Autodesk Inventor part; units mm, degrees
ref_plane "YZ Plane" through (0, 0, 0) normal (1, 0, 0) x (0, 1, 0)
ref_plane "XZ Plane" through (0, 0, 0) normal (0, 1, 0) x (-1, 0, 0)
ref_plane "XY Plane" through (0, 0, 0) normal (0, 0, 1) x (1, 0, 0)
sketch "Sketch1" plane through (0, 0, 0) normal (0, 0, 1) x (1, 0, 0)
  line L0 (0, 88.2) -> (0, -88.2)
  line L1 (-70, 0) -> (70, 0)
  line L2 (-50, -63) -> (50, -63)
  line L3 (50, -63) -> (50, 63)
  line L4 (50, 63) -> (-50, 63)
  line L5 (-50, 63) -> (-50, -63)
  circle A0 centre (0, -20) radius 30
  circle A1 centre (-30, 43) radius 4
  circle A2 centre (30, 43) radius 4
  circle A3 centre (34.8, -54.8) radius 3.25
  circle A4 centre (34.8, 14.8) radius 3.25
  circle A5 centre (-34.8, 14.8) radius 3.25
  circle A6 centre (-34.8, -54.8) radius 3.25
  line L6 (-30, 43) -> (-30, 39)
  line L7 (0, -20) -> (0, 10)
  point P0 (0, 0)
  dimension "d2" = 60
  dimension "d4" = 8
  dimension "d0" = 100
  dimension "d1" = 126
  dimension "d3" = 43
  dimension "d5" = 8
  dimension "d6" = 20
  dimension "d7" = 20
  dimension "d8" = 20
  dimension "d9" = 20
  dimension "d10" = 6.5
  dimension "d11" = 6.5
  dimension "d12" = 6.5
  dimension "d13" = 6.5
  dimension "d14" = 69.6
  dimension "d15" = 69.6
  dimension "d16" = 69.6
  dimension "d17" = 69.6
  dimension "d18" = 0
  dimension "d19" = 0
  dimension "d20" = 34.8
  dimension "d21" = 34.8
  dimension "d22" = 29
extrude "Extrusion1" add sketch "Sketch1" along normal blind 20 contours L4 L3 L1 A0 L0 | L0 A0 L1 L5 L4 | L1 L3 L2 L0 A0 | A0 L0 L2 L5 L1
sketch "Sketch2" plane through (0, 0, 20) normal (0, 0, 1) x (1, 0, 0)
  line L0 (50, 63) -> (-50, 63)
  line L1 (-50, 63) -> (-50, -63)
  line L2 (-50, -63) -> (50, -63)
  line L3 (50, -63) -> (50, 63)
  circle A0 centre (30, 43) radius 4
  circle A1 centre (34.8, 14.8) radius 3.25
  circle A2 centre (34.8, -54.8) radius 3.25
  circle A3 centre (-34.8, -54.8) radius 3.25
  circle A4 centre (-34.8, 14.8) radius 3.25
  circle A5 centre (-30, 43) radius 4
  circle A6 centre (0, -20) radius 30
  line L4 (-50, 63) -> (-50, -63)
  line L5 (-50, 43) -> (50, 43)
  line L6 (-50, 47) -> (50, 47)
  line L7 (-50, 39) -> (50, 39)
  point P0 (0, 0)
  dimension "d25" = 4
  dimension "d26" = 4
extrude "Extrusion2" cut sketch "Sketch2" against normal blind 4 contours L3 L6 L1 L0 | L3 L2 L1 L7
sketch "Sketch3" plane through (0, 0, 0) normal (0, 0, -1) x (-1, 0, 0)
  line L0 (-50, 63) -> (50, 63)
  line L1 (-50, -63) -> (-50, 63)
  line L2 (50, -63) -> (-50, -63)
  line L3 (50, 63) -> (50, -63)
  circle A0 centre (-30, 43) radius 4
  circle A1 centre (-34.8, 14.8) radius 3.25
  circle A2 centre (-34.8, -54.8) radius 3.25
  circle A3 centre (34.8, -54.8) radius 3.25
  circle A4 centre (34.8, 14.8) radius 3.25
  circle A5 centre (30, 43) radius 4
  circle A6 centre (0, -20) radius 30
  point P0 (0, 0)
extrude "Extrusion3" cut sketch "Sketch3" against normal blind 6
properties part number "motor mount lower"
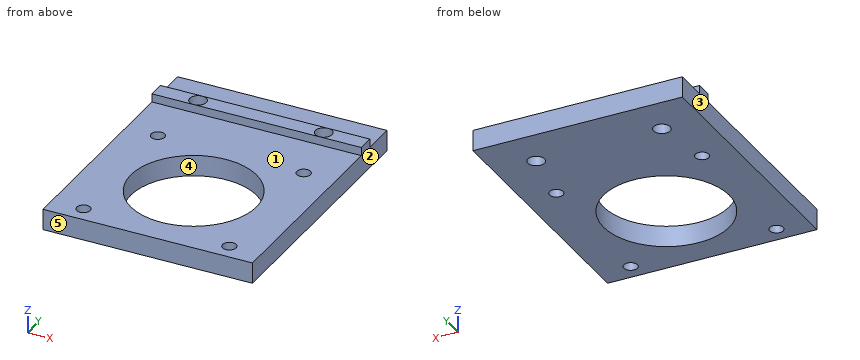
Model file for the job. Use its own axes, mm. Face numbers are marked on the shaded views. A direction names the side the tool comes from. Coordinates: 2 decimals unless noted, no trailing zeros. Write each loop counter-clockwise with the first axis right and the second up, starting at its lowest first coordinate (ties: lowest second). Pieces come first, ordered by that corner, then holes. Notation, with made-up numbers: (-14, 41) -> (44, 41) arc R19 ccw to (44, 78) -> close; hole circle Ø7 at (62, 33.5). An arc over 180 degrees is marked (long way). One line per item, written item: value. Start each with the question number.
1) Slice it at B-B on y = 14.8. Write the cut outline in (x, z), then the cut area to 3 significant figures.
2) Flat gauge pins, fed straight in: pin 1 Ø2 at (x, z) = (-14, 18) entering from -Y; pin 2 Ø6 at (x, y) = (-34.8, 14.8) entering from -Z; pin 3 Ø1.5 at (x, y) = (-10, 22.5) entering from +Z. Where does each tip first touch, or does it go through?
3) Slice it at A-A on z = 8. Write the cut outline in (x, y).
4) Slice it at D-D on y = -20. Write the cut outline in (x, z), then the cut area to 3 significant figures.
5) Slice it at C-C on x = 0. Write the cut outline in (y, z).
6) Pull direction X, two halves, no side cores. Call the marked faces 3, 4 and 5: +X half, -X half, draft (parallel to the pull), parting line (faces both ways), or undercut.
7) Which spindle directions (+Z, -Z, +X, -X, +Y, -Y) get a long thin tool onto all of the face, cutting with end or side? Do the marked faces 1 and 2. Say none if no direction does.
8) Probe probe 1 along Y at (x, z) = (34.8, 10.5); probe 2 along Y at (x, z) = (-27, 14.5); probe 3 along Y at (x, z) = (0, 10.5). List the from-to ranges inside material, lowest first.
Answers follow:
1. outline: (-50, 6) -> (-38.05, 6) -> (-38.05, 16) -> (-50, 16) -> close; (-31.55, 6) -> (31.55, 6) -> (31.55, 16) -> (-31.55, 16) -> close; (38.05, 6) -> (50, 6) -> (50, 16) -> (38.05, 16) -> close
1. area: 870 mm2
2. pin 1: y = 39
2. pin 2: through
2. pin 3: z = 16
3. outline: (-50, -63) -> (50, -63) -> (50, 63) -> (-50, 63) -> close; hole circle Ø6.5 at (-34.8, -54.8); hole circle Ø6.5 at (-34.8, 14.8); hole circle Ø8 at (-30, 43); hole circle Ø60 at (0, -20); hole circle Ø8 at (30, 43); hole circle Ø6.5 at (34.8, -54.8); hole circle Ø6.5 at (34.8, 14.8)
4. outline: (-50, 6) -> (-30, 6) -> (-30, 16) -> (-50, 16) -> close; (30, 6) -> (50, 6) -> (50, 16) -> (30, 16) -> close
4. area: 400 mm2
5. outline: (-63, 6) -> (-50, 6) -> (-50, 16) -> (-63, 16) -> close; (10, 6) -> (63, 6) -> (63, 16) -> (47, 16) -> (47, 20) -> (39, 20) -> (39, 16) -> (10, 16) -> close
6. face 3: -X half
6. face 4: undercut
6. face 5: draft
7. face 1: +Z, +X, -X, -Y
7. face 2: +Z, -Z, +X, +Y, -Y
8. probe 1: -63 to -58.05, -51.55 to 11.55, 18.05 to 63
8. probe 2: -63 to -33.08, -6.92 to 40.35, 45.65 to 63
8. probe 3: -63 to -50, 10 to 63
